Work out the finished part from the listing and answer in its coordinate system (mm). A direction names the side the tool comes from. Coordinates: 2 decimals unless noted, no trailing zeros. Order: outer loops, then holes, each group sorted by start corner. A loop starts at its lowest first (then second) coordinate and runs counter-clockwise, first axis right, second up. Notation, with made-up numbers: (81, 16.5) -> (108, 16.5) arc R17 ccw to (108, 38.5) -> close; hole circle Ø9 at (60, 78.5). An arc over 180 degrees is marked (long way). Write item = value, one per line. Start each with the question number.
Q1. Straight lines are drawn through the part: L1, parallel to Y at x = -49, z = 31; L2, parallel to Z at x = -33, y = -34; L3, parallel to Z at x = -54, y = -23.5. For each, find the intervals that lie inside material, in ascending order. Write a range as from..to.
Q2. Which of the six approach directions +Z, -Z, +X, -X, +Y, -Y give full straight-line access (tool end or side, diameter ignored) to faces 1 (the flat face through (-44, -25.4, 38)), 2 (the flat face through (-29.007, -37.922, 18.692))?
Q3. The part is cut by section A-A, the plane y = -13. Determine the outline of the cut face in (x, z).
Q4. The part is cut by section D-D, the plane x = -28. Determine the outline of the cut face in (y, z), plus the area to 3 significant figures.
Q5. Flat-ended cylindrical pins translate along their axes: pin 1 (1.5 mm diameter, centred on x = -34, z = 18.5, fed in from -Y); pin 2 (20.5 mm diameter, centred on x = -48, y = -41, fed in from +Z); pin 3 (4 mm diameter, centred on x = -47, z = 34.5, fed in from -Y). Find the tip coordinate at first contact, or state that the pin passes through.
Q6. The part is cut by section C-C, the plane z = 17.5. Determine the outline of the cut face in (x, y), plus the area to 3 significant figures.
Q7. The part is cut by section B-B, the plane x = -45.5. Determine the outline of the cut face in (y, z), plus the area to 3 significant figures.
```python
from build123d import *

# Parameters (mm, degrees)
F1_DEPTH = 25.4
F2_W     = 38.1
F2_H     = 12.7
F3_DEPTH = 25.4
F5_DEPTH = 25.4


with BuildPart() as f1:
    # F0 (on Front) → F1 (new body)
    with BuildSketch(Plane.XZ):
        Polygon((-33.318336, 49.470062), (-58.702985, 50.353006), (-58.702985, 12.253006), (-20.602985, 12.253006), (-20.602985, 24.953006), align=None)
    extrude(amount=F1_DEPTH)

    # F2 (on face) → F3 (join)
    with BuildSketch(Plane.XZ.offset(25.4)):
        with Locations((-39.652985, 18.603006)):
            Rectangle(F2_W, F2_H)
    extrude(amount=F3_DEPTH)

    # F4 (on face) → F5 (cut)
    with BuildSketch(Plane.XY.offset(24.953006)):
        Polygon((-20.602985, -50.8), (-20.602985, -25.4), (-37.649736, -50.8), align=None)
    extrude(amount=-F5_DEPTH, mode=Mode.SUBTRACT)


solid = f1.part
```
Model answer:
q1.L1 = -25.4..0
q1.L2 = 12.25..24.95
q1.L3 = 12.25..50.19
q2.face_1 = +Z, +X, -X, -Y
q2.face_2 = +Z, -Z, +X, -Y
q3.outline = (-58.7, 12.25) -> (-20.6, 12.25) -> (-20.6, 24.95) -> (-33.32, 49.47) -> (-58.7, 50.35) -> close
q4.outline = (-36.42, 12.25) -> (0, 12.25) -> (0, 39.22) -> (-25.4, 39.22) -> (-25.4, 24.95) -> (-36.42, 24.95) -> close
q4.area = 825 mm2
q5.pin_1 = -46.48
q5.pin_2 = 24.95
q5.pin_3 = -25.4
q6.outline = (-58.7, -50.8) -> (-37.65, -50.8) -> (-20.6, -25.4) -> (-20.6, 0) -> (-58.7, 0) -> close
q6.area = 1,720 mm2
q7.outline = (-50.8, 12.25) -> (0, 12.25) -> (0, 49.89) -> (-25.4, 49.89) -> (-25.4, 24.95) -> (-50.8, 24.95) -> close
q7.area = 1,280 mm2
